Design review of the part built by this model. Coordinates are the model's own, in mm. A direction names the side the tool comes from. Coordinates: 2 decimals unless noted, no trailing zeros. Loops run counter-clockwise (first coordinate to the right, second up) from the corner with the lowest first, then second, coordinate; pieces in that order, holes last. Notation, with made-up numbers: M -23,44.5 L -10,44.5 A36 ccw -10,82.5 Z; hole C 77,-39.5 d4. An arc over 180 degrees is marked long. Answer as a JSON object with one key per item and string values. Group by question number.
1. Consider section A-A (z = 0). State the section outline as (x, y) points (3 decimals).
2. Draft analysis for pull direction Y (two halves, no side actions). For faces 4 (the cylindrical face through (18.76, -17.37, -36.03)), 5 (the cylindrical face through (18.241, -3.673, 34.623)), 6 (the flat face through (37, 17, 1)), state which applies: +Y half, -Y half, draft (parallel to the pull), parting line (faces both ways), or undercut.
3. Insertion check: pin 1 (1.5 mm diameter, centred on x = 14, y = 21.5, fed in from -Z); pin 2 (3 mm diameter, centred on x = 9, z = 3.5, fed in from +Y); pin 3 (4 mm diameter, centred on x = 17, z = 11, fed in from +Y); pin 4 (19 mm diameter, centred on y = 0, z = 0, fed in from +X). Each pin has a flat end and moves straight along its axis. Give the tip position at first contact, or say it passes through.
4. Consider section C-C (y = -26). State the section outline as (x, z) points, then the cut area to 3 significant figures.
5. Machinability: for faces 1 (the cylindrical face through (18.24, 24.78, 24.46)), 2 (the cylindrical face through (18.24, 11.61, -32.66)), 3 (the cylindrical face through (18.241, 25.886, -12.507)), which of the approach directions +Z, -Z, +X, -X, +Y, -Y give a long, thin tool a straight path to every point of the face, cutting with its end or side? Answer none if there is none.
6. To check wall thickness, follow probe 1 along Y at (x, z) = (17, 0) (3 decimals); probe 2 along Y at (x, z) = (22, 31.5); probe 3 along Y at (x, z) = (13, 35). State the ranges of each line that lie inside material, in increasing order.
7. Consider section D-D (y = 22.5). State the section outline as (x, z) points.
8. Consider section B-B (y = 0). State the section outline as (x, z) points (3 decimals), then the cut area to 3 significant figures.
from build123d import *

# Parameters (mm, degrees)
BASPROSKE_W     = 37
BASPROSKE_H     = 40
TOOTHCUT_DEPTH  = 68.594378464
TEETHCUTS_COUNT = 14
TEETHCUTS_ANGLE = 334.285714286
BORSKE_R        = 15.875
BORE_DEPTH      = 50.000508
CHAMFER1_SIZE   = 0.762


with BuildPart() as part:
    # BasProSke → Base-Revolve (revolve)
    with BuildSketch(Plane(origin=(0, 0, 0), x_dir=(1, 0, 0), z_dir=(0, 1, 0)), mode=Mode.PRIVATE) as base_revolve_sk:
        with Locations((18.5, 20)):
            Rectangle(BASPROSKE_W, BASPROSKE_H)
    revolve(base_revolve_sk.sketch.rotate(Axis((-10, 0, 0), (1, 0, 0)), 180), axis=Axis((-10, 0, 0), (1, 0, 0)))

    # TooCutSke → ToothCut (cut, through all)
    with BuildSketch(Plane(origin=(0, 0, 0), x_dir=(0, 0, -1), z_dir=(1, 0, 0))):
        with BuildLine():
            ThreePointArc((2.668955068, 28.624843752), (0, 28.749), (-2.668955068, 28.624843752))
            ThreePointArc((-2.668955068, 28.624843752), (-4.15928171, 34.644525037), (-8.103646746, 39.429879856))
            ThreePointArc((-8.103646746, 39.429879856), (0, 40.254), (8.103646746, 39.429879856))
            ThreePointArc((8.103646746, 39.429879856), (4.15928171, 34.644525037), (2.668955068, 28.624843752))
        make_face()
    toothcut = extrude(amount=TOOTHCUT_DEPTH, mode=Mode.SUBTRACT)

    # TeethCuts: ToothCut ×14 about axis
    teethcuts_axis = Axis((-10, 0, 0), (1, 0, 0))
    for i in range(1, TEETHCUTS_COUNT):
        add(toothcut.rotate(teethcuts_axis, i * TEETHCUTS_ANGLE / (TEETHCUTS_COUNT - 1)), mode=Mode.SUBTRACT)

    # BorSke → Bore (cut, symmetric)
    with BuildSketch(Plane(origin=(0, 0, 0), x_dir=(0, 0, -1), z_dir=(1, 0, 0))):
        with Locations(Location((0, 0, 0), (0, 0, 180))):
            Circle(BORSKE_R)
    extrude(amount=BORE_DEPTH, both=True, mode=Mode.SUBTRACT)

    # Chamfer1
    chamfer1_edges = [part.edges().sort_by_distance(p)[0] for p in [
        (37, 0, -15.875),
        (0, 0, -15.875),
    ]]
    chamfer(chamfer1_edges, length=CHAMFER1_SIZE)


solid = part.part
Findings below:
{
 "1": {"outline": "M 0,-28.749 L 37,-28.749 L 37,-16.637 L 36.238,-15.875 L 0.762,-15.875 L 0,-16.637 Z; M 0,16.637 L 0.762,15.875 L 36.238,15.875 L 37,16.637 L 37,28.749 L 0,28.749 Z"},
 "2": {"face 4": "-Y half", "face 5": "undercut", "face 6": "draft"},
 "3": {"pin 1": "stops at z = -22.93", "pin 2": "stops at y = 36.09", "pin 3": "stops at y = 38.97", "pin 4": "passes through"},
 "4": {"outline": "M 0,-24.96 L 37,-24.96 L 37,-15.62 L 0,-15.62 Z; M 0,-12.27 L 37,-12.27 L 37,12.27 L 0,12.27 Z; M 0,15.62 L 37,15.62 L 37,24.96 L 0,24.96 Z", "area": "1,600 mm^2"},
 "5": {"face 1": "+Z, +X, -X", "face 2": "-Z, +X, -X", "face 3": "+X, -X"},
 "6": {"probe 1": "y = -28.749 to -15.875, 15.875 to 28.749", "probe 2": "y = -18.61 to -10.78, -4.06 to 4.06, 10.78 to 18.61", "probe 3": "y = -18.43 to -13.98, -3.58 to 3.58, 13.98 to 18.43"},
 "7": {"outline": "M 0,-23.12 L 37,-23.12 L 37,23.12 L 0,23.12 Z"},
 "8": {"outline": "M 0,-40 L 37,-40 L 37,-16.637 L 36.238,-15.875 L 0.762,-15.875 L 0,-16.637 Z; M 0,16.637 L 0.762,15.875 L 36.238,15.875 L 37,16.637 L 37,40 L 0,40 Z", "area": "1,780 mm^2"}
}
